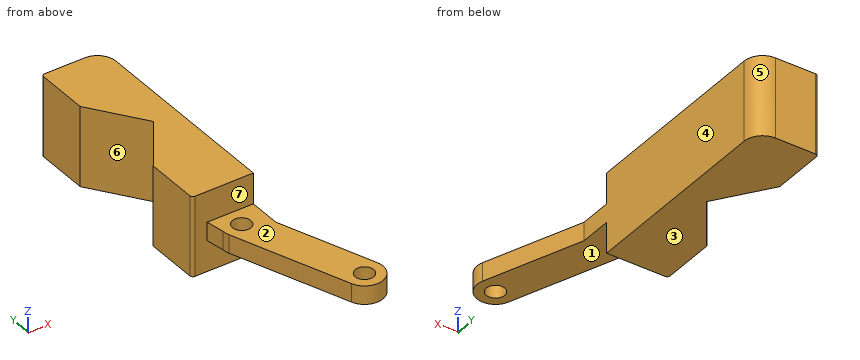
```python
from build123d import *

# Parameters (mm, degrees)
SCHIZZO2_R                        = 1.5
ESTRUSIONE_ESTRUSIONE1_DEPTH      = 1.5
ESTRUSIONE_ESTRUSIONE1_DEPTH_BACK = 1.5
ESTRUSIONE_ESTRUSIONE2_DEPTH      = 6.5
ESTRUSIONE_ESTRUSIONE2_DEPTH_BACK = 6.5
RACCORDO1_R                       = 3
RACCORDO2_R                       = 0.5
RACCORDO3_R                       = 0.5


with BuildPart() as part:
    # Schizzo2 → Estrusione-Estrusione1 (new body, two sides)
    with BuildSketch(Plane.XY) as estrusione_estrusione1_sk:
        with BuildLine():
            Line((2.819077862, 1.02606043), (-4.021325004, 19.819912846))
            ThreePointArc((-4.021325004, 19.819912846), (-7.866463296, 21.612930278), (-9.659480729, 17.767791986))
            Line((-9.659480729, 17.767791986), (-2.819077862, -1.02606043))
            ThreePointArc((-2.819077862, -1.02606043), (1.02606043, -2.819077862), (2.819077862, 1.02606043))
        make_face()
        Circle(SCHIZZO2_R, mode=Mode.SUBTRACT)
        with Locations((-6.840402867, 18.793852416)):
            Circle(SCHIZZO2_R, mode=Mode.SUBTRACT)
        with BuildLine():
            Line((-4.021325004, 19.819912846), (-2.840402867, 16.575355938))
            Line((-2.840402867, 16.575355938), (-2.840402867, 21.793852416))
            Line((-2.840402867, 21.793852416), (-6.840402867, 21.793852416))
            ThreePointArc((-6.840402867, 21.793852416), (-5.119673557, 21.251308549), (-4.021325004, 19.819912846))
        make_face()
        with BuildLine():
            Line((-10.348829971, 21.793852416), (-9.840402867, 18.793852416))
            ThreePointArc((-9.840402867, 18.793852416), (-8.96172321, 20.915172759), (-6.840402867, 21.793852416))
            Line((-6.840402867, 21.793852416), (-10.348829971, 21.793852416))
        make_face()
    extrude(amount=ESTRUSIONE_ESTRUSIONE1_DEPTH)
    extrude(estrusione_estrusione1_sk.sketch, amount=-ESTRUSIONE_ESTRUSIONE1_DEPTH_BACK)

    # Schizzo2_10 → Estrusione-Estrusione2 (add, two sides)
    with BuildSketch(Plane.XY) as estrusione_estrusione2_sk:
        Polygon((-12.840402867, 21.793852416), (-10.348829971, 21.793852416), (-6.840402867, 21.793852416), (-2.840402867, 21.793852416), (-2.840402867, 56.793852416), (-12.840402867, 56.793852416), (-12.840402867, 47.793852416), (-6.840402867, 39.293852416), (-12.840402867, 30.793852416), align=None)
    extrude(amount=ESTRUSIONE_ESTRUSIONE2_DEPTH)
    extrude(estrusione_estrusione2_sk.sketch, amount=-ESTRUSIONE_ESTRUSIONE2_DEPTH_BACK)

    # Raccordo1
    raccordo1_edges = [part.edges().sort_by_distance(p)[0] for p in [
        (-2.840402867, 56.793852416, 0),
    ]]
    fillet(raccordo1_edges, radius=RACCORDO1_R)

    # Raccordo2
    raccordo2_edges = [part.edges().sort_by_distance(p)[0] for p in [
        (-12.840402867, 21.793852416, 0),
    ]]
    fillet(raccordo2_edges, radius=RACCORDO2_R)

    # Raccordo3
    raccordo3_edges = [part.edges().sort_by_distance(p)[0] for p in [
        (-12.840402867, 56.793852416, 0),
    ]]
    fillet(raccordo3_edges, radius=RACCORDO3_R)


solid = part.part
```
The model under review builds one solid part; all positions refer to its coordinate system, in mm. Face numbers are marked on the shaded views. A direction names the side the tool comes from. Round coordinates to 2 decimals unless told otherwise and drop trailing zeros. Order: outer loops, then holes, each group sorted by start corner. A loop starts at its lowest first (then second) coordinate and runs counter-clockwise, first axis right, second up. Notation, with made-up numbers: (61, -21.5) -> (96, -21.5) arc R12 ccw to (96, -1.5) -> close; hole circle Ø5 at (72, 30). An arc over 180 degrees is marked (long way). Use a Markdown table: item, result.
Q1. Clearance check with flat-ended pins moving along their axes: P1, Ø1, axis at x = -4, y = 11.5, coming from the +Z side; P2, Ø1, axis at x = -3.5, z = -2.5, coming from the -Y side; P3, Ø4, axis at y = 32.5, z = 0, coming from the +X side. State where each tip first meets the part, or that it passes through.
Values:
| item | result |
|---|---|
| P1 | stops at z = 1.5 |
| P2 | stops at y = 21.79 |
| P3 | stops at x = -2.84 |
Q2. For line 1 (Y direction, x = -10.75, z = -1.25); line 2 (X direction, y = 52, z = -5); line 3 (Y direction, x = -9.75, z = 2), list the stretches that pass through material, from the lowest coordinate up.
Values:
| item | result |
|---|---|
| line 1 | y = 21.79 to 33.76, 44.83 to 56.79 |
| line 2 | x = -12.84 to -2.84 |
| line 3 | y = 21.79 to 35.17, 43.42 to 56.79 |
Q3. Tool access review of the marked faces 1, 2, 3 and 4: name each direction out of +Z, -Z, +X, -X, +Y, -Y from which nothing blocks a thin tool from reaching the whole face with its end or side.
Values:
| item | result |
|---|---|
| face 1 | -Z, +X, -X, -Y |
| face 2 | +Z, +X, -X, -Y |
| face 3 | -Z, +X, -X, +Y, -Y |
| face 4 | +Z, -Z, +X, +Y |
Q4. Mouldability with a two-part tool opening along Y and no side actions: class the marked faces 5, 6 and 7 as +Y half, -Y half, draft (parallel to the pull), parting line (faces both ways), or undercut.
Values:
| item | result |
|---|---|
| face 5 | +Y half |
| face 6 | undercut |
| face 7 | -Y half |
Q5. We need section C-C on x = -0.25. Write out the cut boundary in (y, z).
Values:
| item | result |
|---|---|
| outline | (-2.99, -1.5) -> (-1.48, -1.5) -> (-1.48, 1.5) -> (-2.99, 1.5) -> close; (1.48, -1.5) -> (9.46, -1.5) -> (9.46, 1.5) -> (1.48, 1.5) -> close |
Q6. We need section B-B on y = 0. Write out the cut boundary in (x, z), then the cut area to 3 significant figures.
Values:
| item | result |
|---|---|
| outline | (-3.19, -1.5) -> (-1.5, -1.5) -> (-1.5, 1.5) -> (-3.19, 1.5) -> close; (1.5, -1.5) -> (3, -1.5) -> (3, 1.5) -> (1.5, 1.5) -> close |
| area | 9.58 mm^2 |
Q7. We need section A-A on z = -0.75. Write out the cut boundary in (x, y), then the cut area to 3 significant figures.
Values:
| item | result |
|---|---|
| outline | (-12.84, 22.29) arc R0.5 ccw to (-12.34, 21.79) -> (-10.35, 21.79) -> (-9.84, 18.79) arc R3 ccw to (-9.66, 17.77) -> (-2.82, -1.03) arc R3 ccw to (2.82, 1.03) -> (-2.84, 16.58) -> (-2.84, 53.79) arc R3 ccw to (-5.84, 56.79) -> (-12.34, 56.79) arc R0.5 ccw to (-12.84, 56.29) -> (-12.84, 47.79) -> (-6.84, 39.29) -> (-12.84, 30.79) -> close; hole circle Ø3 at (-6.84, 18.79); hole circle Ø3 at (0, 0) |
| area | 440 mm^2 |
Q8. We need section D-D on z = 5.5. Write out the cut boundary in (x, y), then the cut area to 3 significant figures.
Values:
| item | result |
|---|---|
| outline | (-12.84, 22.29) arc R0.5 ccw to (-12.34, 21.79) -> (-2.84, 21.79) -> (-2.84, 53.79) arc R3 ccw to (-5.84, 56.79) -> (-12.34, 56.79) arc R0.5 ccw to (-12.84, 56.29) -> (-12.84, 47.79) -> (-6.84, 39.29) -> (-12.84, 30.79) -> close |
| area | 297 mm^2 |
